For this review, take the finished solid that the model builds, in its own axes (mm). Give positions to 0.01 mm unless a question says otherwise; leave off trailing zeros. Loops run counter-clockwise (first coordinate to the right, second up) from the corner with the lowest first, then second, coordinate; pieces in that order, holes last.
Autodesk Inventor part; units mm, degrees
ref_plane "YZ Plane" through (0, 0, 0) normal (1, 0, 0) x (0, 1, 0)
ref_plane "XZ Plane" through (0, 0, 0) normal (0, 1, 0) x (-1, 0, 0)
ref_plane "XY Plane" through (0, 0, 0) normal (0, 0, 1) x (1, 0, 0)
sketch "Sketch1" plane through (0, 0, 0) normal (0, 0, 1) x (1, 0, 0)
  line L0 (0, 0) -> (89.154, 0)
  line L1 (89.154, 0) -> (89.154, 17.78)
  line L2 (89.154, 17.78) -> (0, 17.78)
  line L3 (0, 17.78) -> (0, 0)
  dimension "d0" = 89.154
  dimension "d1" = 17.78
extrude "Extrusion1" add sketch "Sketch1" along normal blind 10.16
sketch "Sketch2" plane through (0, 0, 10.16) normal (0, 0, 1) x (1, 0, 0)
  line L0 (0, 17.78) -> (0, 0)
  line L1 (0, 0) -> (89.154, 0)
  point P0 (19.05, 2.54)
  point P1 (69.85, 2.54)
  point P2 (0, 8.89)
  dimension "d4" = 19.05
  dimension "d5" = 50.8
  dimension "d6" = 2.54
hole "Hole1" at (19.05, 2.54, 10.16) at (69.85, 2.54, 10.16) direction (0, 0, -1) diameter 2.667 end through all
properties part number "Coupler"
Q1. For pin 1 Ø2.5 at (x, y) = (19.05, 2.54) entering from +Z, flat-tipped, find the tip position at first contact; note if it passes through.
Answers:
pin 1: passes through
Q2. For probe 1 along Y at (x, z) = (69.85, 6.75); probe 2 along X at (y, z) = (2.54, 3); probe 3 along X at (y, z) = (3, 4.5), list the stretches that pass through material, from the lowest coordinate up.
Answers:
probe 1: y = 0 to 1.21, 3.87 to 17.78
probe 2: x = 0 to 17.72, 20.38 to 68.52, 71.18 to 89.15
probe 3: x = 0 to 17.8, 20.3 to 68.6, 71.1 to 89.15
Q3. Mouldability with a two-part tool opening along Y and no side actions: class faces 1 (the flat face through (45, 17.78, 5)), 2 (the flat face through (44, 0, 5)), 3 (the cylindrical face through (68.949, 3.523, 5.009)), 4 (the flat face through (89.154, 9, 5)) as +Y half, -Y half, draft (parallel to the pull), parting line (faces both ways), or undercut.
Answers:
face 1: +Y half
face 2: -Y half
face 3: undercut
face 4: draft
Q4. Consider section A-A on x = 69.85. Give the boundary of the cut face in (y, z).
Answers:
outline: (0, 0) - (1.21, 0) - (1.21, 10.16) - (0, 10.16) - close; (3.87, 0) - (17.78, 0) - (17.78, 10.16) - (3.87, 10.16) - close
